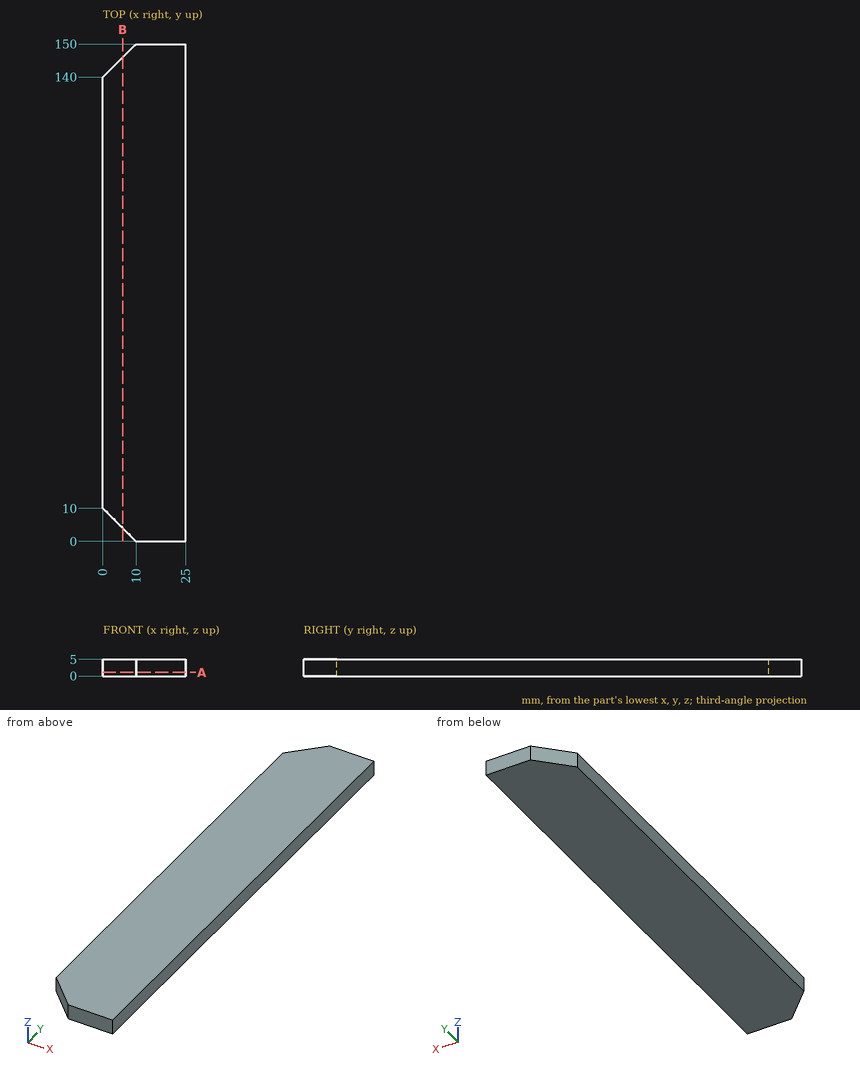
Could you check a few things on this drawing? It's one solid part, dimensions in mm from its lowest x, y, z. Coordinates: 2 decimals unless noted, no trailing zeros. Write each loop counter-clockwise with the first axis right and the second up, starting at its lowest first coordinate (ties: lowest second). Pieces come first, ordered by that corner, then holes. Notation, with made-up numbers: (43.25, 47) - (62.25, 47) arc R12 ccw to (62.25, 58) - close; hole circle Ø10 at (23.5, -12). An arc over 180 degrees is marked (long way). Use one line per item in the form item = value.
1) I'm going to push a flat-ended pin straight in: P1, Ø3, axis at x = 7, z = 2, coming from the +Y side. Where does the tip first touch, or does it pass through?
Solved:
P1 = 148.5
2) Suppose I cut it at A-A, the plane z = 1.1. Write out the boundary of the cut face in (x, y), plus the area to 3 significant figures.
Solved:
outline = (0, 10) - (10, 0) - (25, 0) - (25, 150) - (10, 150) - (0, 140) - close
area = 3,650 mm2
3) I need wall thicknesses on line 1 (Y direction, x = 4.25, z = 2.4); line 2 (Y direction, x = 7, z = 3.5); line 3 (X direction, y = 6, z = 4.2). Which ranges of each line are inside material? Lowest first, please.
Solved:
line_1 = 5.75 to 144.25
line_2 = 3 to 147
line_3 = 4 to 25
4) Suppose I cut it at B-B, the plane x = 6. Write out the boundary of the cut face in (y, z), plus the area to 3 significant figures.
Solved:
outline = (4, 0) - (146, 0) - (146, 5) - (4, 5) - close
area = 710 mm2
